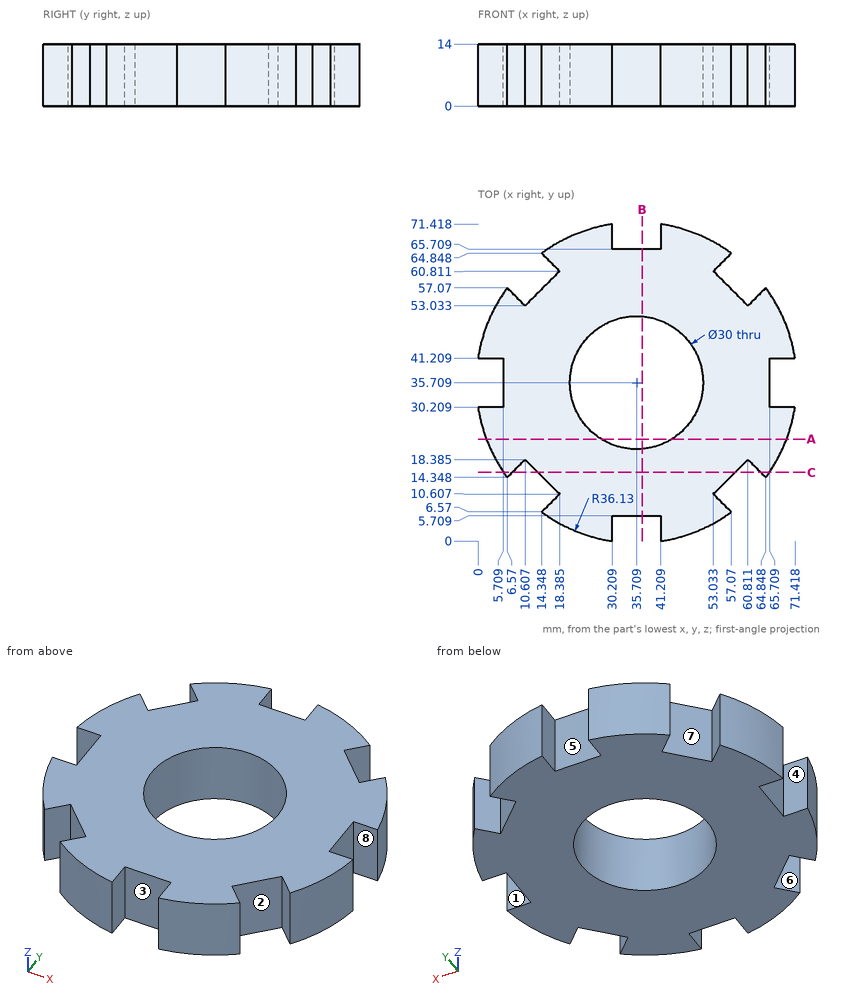
Design review of the part shown in the three views and the two pictorial views. Dimensions are in mm from the part's minimum x, y and z. A direction names the side the tool comes from. Round coordinates to 2 decimals unless told otherwise and drop trailing zeros. Loops run counter-clockwise (first coordinate to the right, second up) from the corner with the lowest first, then second, coordinate; pieces in that order, holes last. Notation, with made-up numbers: M 56,21.25 L 92,21.25 A32 ccw 92,50.25 Z; hole C 11,18.5 d6. An arc over 180 degrees is marked long. Answer as a JSON object with one key per item and string values.
Item 1: We need section C-C on y = 15.5. Give the boundary of the cut face in (x, z).
Answer sheet:
{"outline": "M 5.76,0 L 7.72,0 L 7.72,14 L 5.76,14 Z; M 13.49,0 L 57.93,0 L 57.93,14 L 13.49,14 Z; M 63.7,0 L 65.66,0 L 65.66,14 L 63.7,14 Z"}
Item 2: Machinability: for the marked faces 1, 2, 3 and 4, which of the approach directions +Z, -Z, +X, -X, +Y, -Y give a long, thin tool a straight path to every point of the face, cutting with its end or side? Answer none if there is none.
Answer sheet:
{"face 1": "+Z, -Z, +X", "face 2": "+Z, -Z", "face 3": "+Z, -Z, -Y", "face 4": "+Z, -Z, -X"}
Item 3: We need section B-B on x = 37. Give the boundary of the cut face in (y, z) (1 decimal).
Answer sheet:
{"outline": "M 5.7,0 L 20.8,0 L 20.8,14 L 5.7,14 Z; M 50.7,0 L 65.7,0 L 65.7,14 L 50.7,14 Z"}
Item 4: We need section A-A on y = 23. Give the boundary of the cut face in (x, z).
Answer sheet:
{"outline": "M 1.89,0 L 27.74,0 L 27.74,14 L 1.89,14 Z; M 43.68,0 L 69.53,0 L 69.53,14 L 43.68,14 Z"}
Item 5: The part is to be moulded in two halves that separate along X. For the marked faces 5, 6, 7 and 8, say which applies: pulls with the +X half, pulls with the -X half, needs draft (parallel to the pull), parting line crosses it, or undercut.
Answer sheet:
{"face 5": "undercut", "face 6": "pulls with the -X half", "face 7": "undercut", "face 8": "needs draft"}
Item 6: Clearance check with flat-ended pins moving along their axes: P1, Ø4.5, axis at y = 1.5, z = 6.5, coming from the +X side; P2, Ø3, axis at x = 69.5, z = 9.5, coming from the +Y side (1 decimal); P3, Ø1, axis at y = 32, z = 11, coming from the -X side. State where each tip first meets the part, or that it passes through.
Answer sheet:
{"P1": "stops at x = 52.56", "P2": "stops at y = 51.9", "P3": "stops at x = 5.71"}
Item 7: Wall thickness on L1, parallel to Y at x = 16, z = 10 (1 decimal); L2, parallel to Y at x = 53.5, z = 2.25 (1 decimal); L3, parallel to Y at x = 48, z = 3 (1 decimal): over which ranges is each line inside the solid? List them lowest first. Write a range as from..to.
Answer sheet:
{"L1": "y = 5.4..8.2, 13..58.4, 63.2..66", "L2": "y = 4.3..10.1, 11.1..60.3, 61.3..67.2", "L3": "y = 1.7..27.1, 44.3..69.7"}
